Could you check a few things on this drawing? It's one solid part, dimensions in mm from its lowest x, y, z. A direction names the side the tool comes from. Coordinates: 2 decimals unless noted, no trailing zeros. Write each loop counter-clockwise with the first axis right and the second up, starting at its lowest first coordinate (ties: lowest second). Pieces come first, ordered by that corner, then holes. Notation, with made-up numbers: M -34,-1.75 L -22,-1.75 A15 cw -22,20.25 Z; hole C 15,37 d11. An arc over 180 degrees is marked long. Use a Markdown table: item, result.
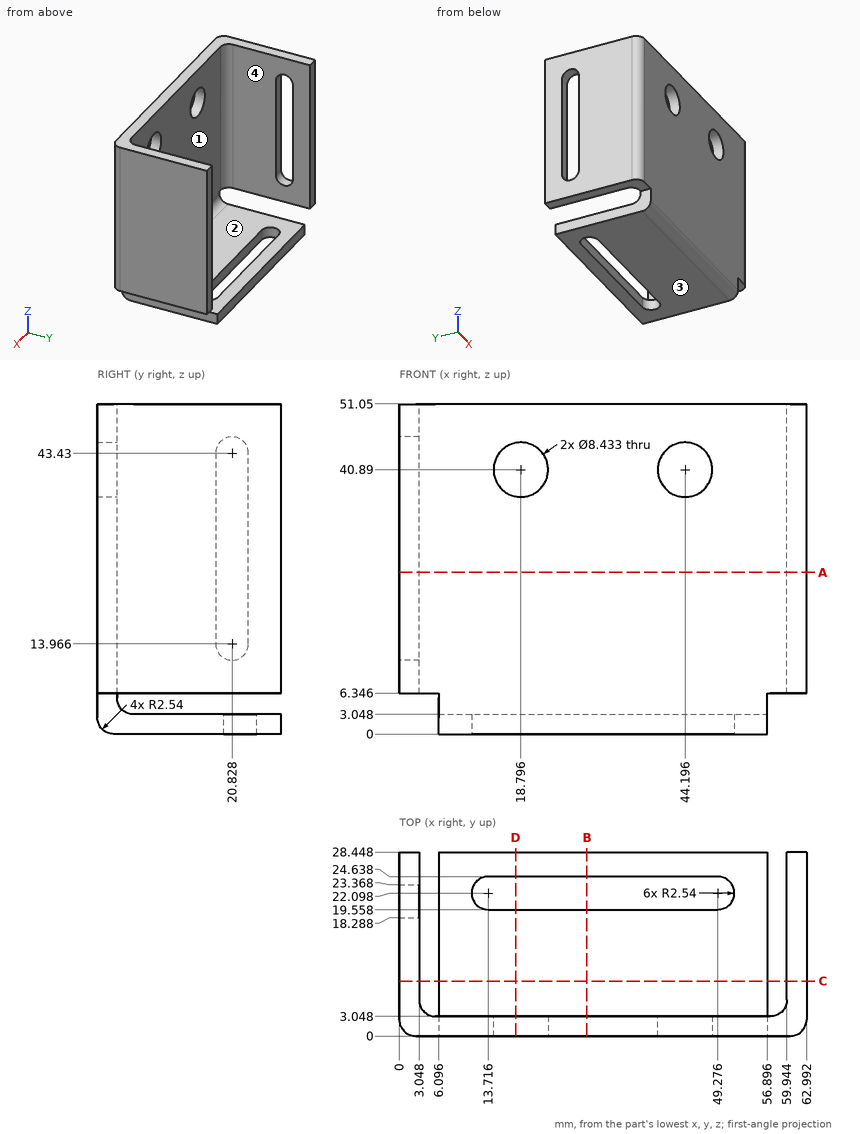
1. Suppose I cut it at D-D on x = 18. Write out the boundary of the cut face in (y, z).
Answers follow:
| item | result |
|---|---|
| outline | M 0,2.54 A2.54 ccw 2.54,0 L 19.56,0 L 19.56,3.05 L 5.59,3.05 A2.54 cw 3.05,5.59 L 3.05,36.75 L 0,36.75 Z; M 0,45.03 L 3.05,45.03 L 3.05,51.05 L 0,51.05 Z; M 24.64,0 L 28.45,0 L 28.45,3.05 L 24.64,3.05 Z |
2. Suppose I cut it at A-A on z = 25. Write out the boundary of the cut face in (x, y), and give its area (3 significant figures).
Answers follow:
| item | result |
|---|---|
| outline | M 0,2.54 A2.54 ccw 2.54,0 L 60.45,0 A2.54 ccw 62.99,2.54 L 62.99,28.45 L 59.94,28.45 L 59.94,5.59 A2.54 cw 57.4,3.05 L 5.59,3.05 A2.54 cw 3.05,5.59 L 3.05,18.29 L 0,18.29 Z; M 0,23.37 L 3.05,23.37 L 3.05,28.45 L 0,28.45 Z |
| area | 331 mm2 |
3. Will these pins go through, and if not, where does the flat tip stop? pin 1 Ø2.5 at (x, z) = (1, 21.5) entering from -Y; pin 2 Ø22.5 at (x, z) = (30.5, 17) entering from +Y; pin 3 Ø6 at (y, z) = (17.5, 43.5) entering from -X; pin 4 Ø1.8 at (x, y) = (1.5, 7) entering from -Z.
Answers follow:
| item | result |
|---|---|
| pin 1 | stops at y = 0.02 |
| pin 2 | stops at y = 3.05 |
| pin 3 | stops at x = 0 |
| pin 4 | stops at z = 6.35 |
4. I need wall thicknesses on probe 1 along X at (y, z) = (12, 12); probe 2 along Y at (x, z) = (48.5, 3); probe 3 along X at (y, z) = (2.75, 5). Which ranges of each line are inside material? Lowest first, please.
Answers follow:
| item | result |
|---|---|
| probe 1 | x = 0 to 3.05, 59.94 to 62.99 |
| probe 2 | y = 0 to 19.56, 24.64 to 28.45 |
| probe 3 | x = 6.1 to 56.9 |
5. Suppose I cut it at C-C on y = 8.5. Write out the boundary of the cut face in (x, z).
Answers follow:
| item | result |
|---|---|
| outline | M 0,6.35 L 3.05,6.35 L 3.05,51.05 L 0,51.05 Z; M 6.1,0 L 56.9,0 L 56.9,3.05 L 6.1,3.05 Z; M 59.94,6.35 L 62.99,6.35 L 62.99,51.05 L 59.94,51.05 Z |
6. Suppose I cut it at B-B on x = 29. Write out the boundary of the cut face in (y, z).
Answers follow:
| item | result |
|---|---|
| outline | M 0,2.54 A2.54 ccw 2.54,0 L 19.56,0 L 19.56,3.05 L 5.59,3.05 A2.54 cw 3.05,5.59 L 3.05,51.05 L 0,51.05 Z; M 24.64,0 L 28.45,0 L 28.45,3.05 L 24.64,3.05 Z |
7. Which directions (+Z, -Z, +X, -X, +Y, -Y) give clear straight access to the entire face, cutting with the end or side of a thin tool? Please do the marked faces 1, 2, 3 and 4.
Answers follow:
| item | result |
|---|---|
| face 1 | +Z, +Y |
| face 2 | +Z, +X, -X, +Y |
| face 3 | -Z, +X, -X, +Y, -Y |
| face 4 | +Z, -Z, +Y |
